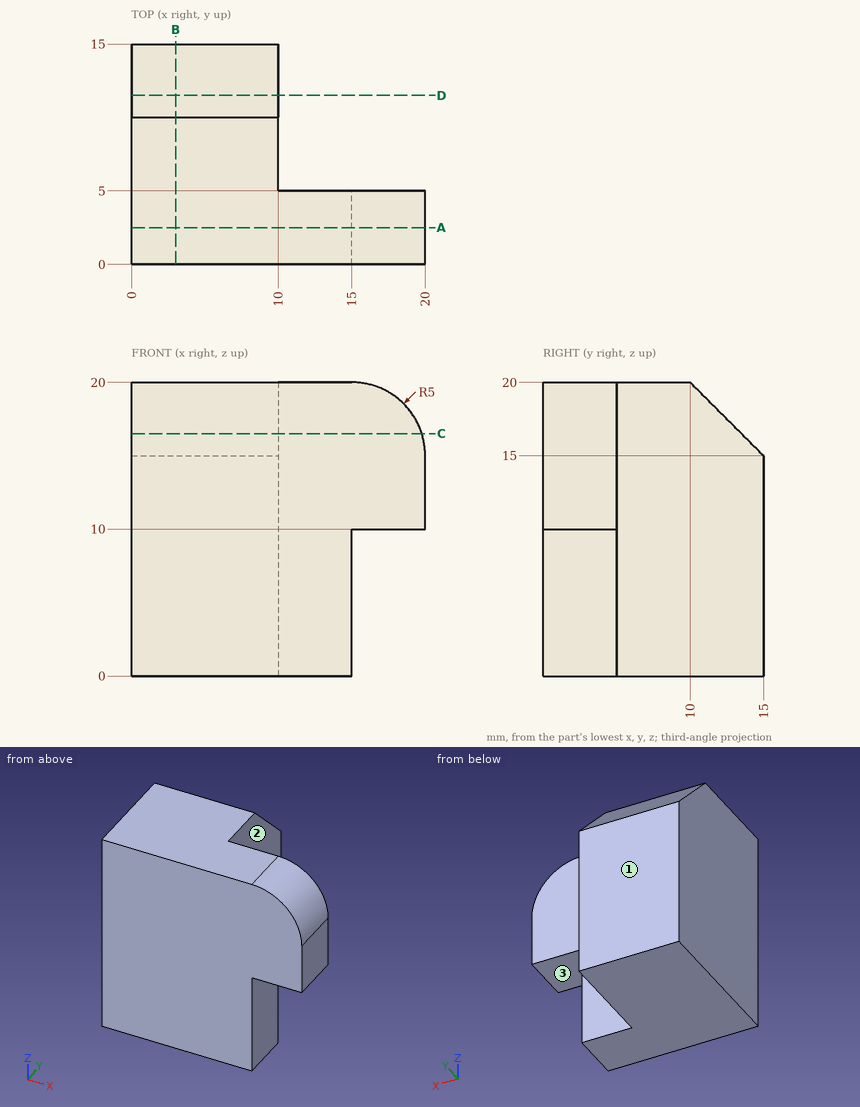
Drawing for the job (mm, zero at the part's lowest x, y, z). A direction names the side the tool comes from. Give positions to 0.01 mm unless a question says otherwise; leave off trailing zeros. Order: outer loops, then holes, each group sorted by start corner. A loop starts at its lowest first (then second) coordinate and runs counter-clockwise, first axis right, second up. Notation, with made-up numbers: M -26.5,-19 L -22.5,-19 A29 cw -22.5,10 Z; hole C 17,78.25 d7. An arc over 180 degrees is marked long. Write item = value, one per line. Start each with the question number.
(1) Which spindle directions (+Z, -Z, +X, -X, +Y, -Y) get a long thin tool onto all of the face, cutting with end or side? Do the marked faces 1, 2 and 3. Say none if no direction does.
(2) Slice it at D-D on y = 11.5. Write the cut outline in (x, z), plus the area to 3 significant figures.
(3) Pin check, flat tips, straight feed: pin 1 Ø5 at (y, z) = (11.5, 11) entering from +X; pin 2 Ø4 at (y, z) = (2.5, 5.5) entering from +X; pin 3 Ø4 at (x, y) = (18.5, 1.5) entering from -Z. Stop position of each tip, or through.
(4) Slice it at A-A on y = 2.5. Write the cut outline in (x, z).
(5) Slice it at C-C on z = 16.5. Write the cut outline in (x, y), plus the area to 3 significant figures.
(6) Slice it at B-B on x = 3. Write the cut outline in (y, z), plus the area to 4 significant figures.
(7) Probe L1, parallel to X at y = 13, z = 5.5; L2, parallel to X at y = 1, z = 4.5; L3, parallel to Y at x = 12.5, z = 10.75. List the from-to ranges inside material, lowest first. Write a range as [from, to].
Responses:
q1.face_1 = +Z, -Z, +X, -X, +Y
q1.face_2 = +Z, -Z, +X, +Y
q1.face_3 = -Z, +X, +Y, -Y
q2.outline = M 0,0 L 10,0 L 10,18.5 L 0,18.5 Z
q2.area = 185 mm2
q3.pin_1 = 10
q3.pin_2 = 15
q3.pin_3 = 10
q4.outline = M 0,0 L 15,0 L 15,10 L 20,10 L 20,15 A5 ccw 15,20 L 0,20 Z
q5.outline = M 0,0 L 19.77,0 L 19.77,5 L 10,5 L 10,13.5 L 0,13.5 Z
q5.area = 184 mm2
q6.outline = M 0,0 L 15,0 L 15,15 L 10,20 L 0,20 Z
q6.area = 287.5 mm2
q7.L1 = [0, 10]
q7.L2 = [0, 15]
q7.L3 = [0, 5]
